The listing builds one solid part. Answer for the finished solid, in the listing's coordinates (mm). A direction names the side the tool comes from. Coordinates: 2 decimals unless noted, no trailing zeros.
from build123d import *

# Parameters (mm, degrees)
SKETCH4_R           = 2.65
SKETCH4_R_2         = 8
BOSS_EXTRUDE1_DEPTH = 5


with BuildPart() as part:
    # Sketch4 → Boss-Extrude1 (new body)
    with BuildSketch(Plane.XY):
        with BuildLine():
            Line((-115.538340842, -75), (115.538340842, -75))
            add(Edge.make_bspline(
                [(115.538340842, -75), (157.739845208, 0), (115.538340842, 75)],
                knots=[1.027171819, 1.027171819, 1.027171819, 2.114420834, 2.114420834, 2.114420834], degree=2, weights=[1, 0.855839562, 1]))
            Line((115.538340842, 75), (-115.538340842, 75))
            add(Edge.make_bspline(
                [(-115.538340842, 75), (-157.739845208, 0), (-115.538340842, -75)],
                knots=[4.168764473, 4.168764473, 4.168764473, 5.256013488, 5.256013488, 5.256013488], degree=2, weights=[1, 0.855839562, 1]))
        make_face()
        with Locations((0, 35)):
            Circle(SKETCH4_R, mode=Mode.SUBTRACT)
        with Locations((30.310889132, 17.5)):
            Circle(SKETCH4_R, mode=Mode.SUBTRACT)
        with Locations((30.310889132, -17.5)):
            Circle(SKETCH4_R, mode=Mode.SUBTRACT)
        with Locations((0, -35)):
            Circle(SKETCH4_R, mode=Mode.SUBTRACT)
        with Locations((-30.310889132, -17.5)):
            Circle(SKETCH4_R, mode=Mode.SUBTRACT)
        with Locations((-30.310889132, 17.5)):
            Circle(SKETCH4_R, mode=Mode.SUBTRACT)
        with Locations((64.752033934, 17.5)):
            Circle(SKETCH4_R_2, mode=Mode.SUBTRACT)
        with Locations((74.374721355, 44.185460771)):
            Circle(SKETCH4_R_2, mode=Mode.SUBTRACT)
        with Locations((99.888536583, 59.516130447)):
            Circle(SKETCH4_R_2, mode=Mode.SUBTRACT)
        with Locations(Location((-99.888536583, 59.516130447, 0), (0, 0, 180))):
            Circle(SKETCH4_R_2, mode=Mode.SUBTRACT)
        with Locations(Location((-74.374721355, 44.185460771, 0), (0, 0, 180))):
            Circle(SKETCH4_R_2, mode=Mode.SUBTRACT)
        with Locations(Location((-64.752033934, 17.5, 0), (0, 0, 180))):
            Circle(SKETCH4_R_2, mode=Mode.SUBTRACT)
        with Locations((120.644049354, -38.948255584)):
            Circle(SKETCH4_R, mode=Mode.SUBTRACT)
        with Locations((122.664887702, 29.201114123)):
            Circle(SKETCH4_R, mode=Mode.SUBTRACT)
        with Locations(Location((-122.664887702, 29.201114123, 0), (0, 0, 180))):
            Circle(SKETCH4_R, mode=Mode.SUBTRACT)
        with Locations(Location((-120.644049354, -38.948255584, 0), (0, 0, 180))):
            Circle(SKETCH4_R, mode=Mode.SUBTRACT)
        with BuildLine():
            Line((96.221427668, -66.569190125), (24.443369148, -42.131459749))
            ThreePointArc((24.443369148, -42.131459749), (21.104097738, -38.098339283), (23.194170579, -33.297465429))
            Line((23.194170579, -33.297465429), (31.044827796, -27.820928801))
            ThreePointArc((31.044827796, -27.820928801), (36.634624949, -21.900779304), (39.401541781, -14.243222677))
            Line((39.401541781, -14.243222677), (40.142546192, -9.050682376))
            ThreePointArc((40.142546192, -9.050682376), (41.921887066, -5.890808111), (45.369026009, -4.764712013))
            Line((45.369026009, -4.764712013), (111.686928814, -8.439409623))
            ThreePointArc((111.686928814, -8.439409623), (115.232710002, -10.208524402), (116.377662166, -14.002126368))
            add(Edge.make_bspline(
                [(116.377662166, -14.002126368), (115.220834159, -24.076872303), (111.675987444, -41.055400313), (105.466013317, -57.243285168), (102.371009367, -63.934943838)],
                knots=[0.084665499, 0.084665499, 0.084665499, 0.084665499, 0.572063361, 0.927683596, 0.927683596, 0.927683596, 0.927683596], degree=3))
            ThreePointArc((102.371009367, -63.934943838), (99.801685805, -66.432067651), (96.221427668, -66.569190125))
        make_face(mode=Mode.SUBTRACT)
        with BuildLine():
            Line((115.869646859, 8.131830129), (111.070686254, 37.070959775))
            ThreePointArc((111.070686254, 37.070959775), (109.047553267, 40.319281474), (105.320071912, 41.18562072))
            Line((105.320071912, 41.18562072), (94.654082301, 39.416885289))
            ThreePointArc((94.654082301, 39.416885289), (92.149315195, 38.220472158), (90.668652636, 35.872515381))
            Line((90.668652636, 35.872515381), (83.183473525, 9.973795657))
            ThreePointArc((83.183473525, 9.973795657), (83.908923245, 5.692386099), (87.710252524, 3.593186057))
            Line((87.710252524, 3.593186057), (110.66038185, 2.321511565))
            ThreePointArc((110.66038185, 2.321511565), (114.659851997, 3.97612342), (115.869646859, 8.131830129))
        make_face(mode=Mode.SUBTRACT)
        with BuildLine():
            Line((-96.221427668, -66.569190125), (-24.443369148, -42.131459749))
            ThreePointArc((-24.443369148, -42.131459749), (-21.104097738, -38.098339283), (-23.194170579, -33.297465429))
            Line((-23.194170579, -33.297465429), (-31.044827796, -27.820928801))
            ThreePointArc((-31.044827796, -27.820928801), (-36.634624949, -21.900779304), (-39.401541781, -14.243222677))
            Line((-39.401541781, -14.243222677), (-40.142546192, -9.050682376))
            ThreePointArc((-40.142546192, -9.050682376), (-41.921887066, -5.890808111), (-45.369026009, -4.764712013))
            Line((-45.369026009, -4.764712013), (-111.686928814, -8.439409623))
            ThreePointArc((-111.686928814, -8.439409623), (-115.232710002, -10.208524402), (-116.377662166, -14.002126368))
            add(Edge.make_bspline(
                [(-116.377662166, -14.002126368), (-115.220834159, -24.076872303), (-111.675987444, -41.055400313), (-105.466013317, -57.243285168), (-102.371009367, -63.934943838)],
                knots=[0.084665499, 0.084665499, 0.084665499, 0.084665499, 0.572063361, 0.927683596, 0.927683596, 0.927683596, 0.927683596], degree=3))
            ThreePointArc((-102.371009367, -63.934943838), (-99.801685805, -66.432067651), (-96.221427668, -66.569190125))
        make_face(mode=Mode.SUBTRACT)
        with BuildLine():
            Line((-90.668652636, 35.872515381), (-83.183473525, 9.973795657))
            ThreePointArc((-83.183473525, 9.973795657), (-83.908923245, 5.692386099), (-87.710252524, 3.593186057))
            Line((-87.710252524, 3.593186057), (-110.66038185, 2.321511565))
            ThreePointArc((-110.66038185, 2.321511565), (-114.659851997, 3.97612342), (-115.869646859, 8.131830129))
            Line((-115.869646859, 8.131830129), (-111.070686254, 37.070959775))
            ThreePointArc((-111.070686254, 37.070959775), (-109.047553267, 40.319281474), (-105.320071912, 41.18562072))
            Line((-105.320071912, 41.18562072), (-94.654082301, 39.416885289))
            ThreePointArc((-94.654082301, 39.416885289), (-92.149315195, 38.220472158), (-90.668652636, 35.872515381))
        make_face(mode=Mode.SUBTRACT)
    extrude(amount=BOSS_EXTRUDE1_DEPTH)


solid = part.part
Q1. Given pin 1 (2 mm diameter, centred on y = -49.5, z = 4, fed in from +X); pin 2 (4 mm diameter, centred on x = 0.5, y = -59.5, fed in from -Z); pin 3 (3 mm diameter, centred on y = -16.5, z = 2, fed in from +X), each flat-ended and moving along its own axis, determine where each tip first touches the part or whether it passes through.
Answers below:
pin 1: stops at x = 127.22
pin 2: stops at z = 0
pin 3: stops at x = 134.28
Q2. The part is cut by section A-A, the plane y = 56.5. State how many separate pieces and enclosed holes the cut face has, then the cut area to 3 significant figures.
Answers below:
separate pieces: 3
enclosed holes: 0
area: 1,100 mm2
Q3. Find the intervals of material crossed by probe 1 along X at (y, z) = (48, 4.7); probe 2 along Y at (x, z) = (-61, 4.05); probe 3 along X at (y, z) = (-42, 1.05), in increasing order.
Answers below:
probe 1: x = -127.39 to -81.41, -67.34 to 67.34, 81.41 to 127.39
probe 2: y = -75 to -54.58, -5.63 to 10.43, 24.57 to 75
probe 3: x = -129.21 to -110.67, -24.1 to 24.1, 110.67 to 129.21
Q4. Which of the six approach directions +Z, -Z, +X, -X, +Y, -Y give full straight-line access (tool end or side, diameter ignored) to faces 4 (the face through (-2, 1, 0)), 5 (the face through (36.574, -21.998, 2.465))?
Answers below:
face 4: -Z, +X, -X, +Y, -Y
face 5: +Z, -Z
Q5. Determine the mould class of faces 1 (the face through (-86.978, 23.104, 2.465)), 2 (the face through (27.06, -30.6, 2.46)), 3 (the face through (2, 75, 2)) for opening direction X: released by +X, released by -X, zero draft, split by the parting line, or undercut.
Answers below:
face 1: undercut
face 2: undercut
face 3: zero draft
